Source: CAD feature listing. Evaluate the final solid. Frame: model axes, mm. Face numbers are marked on the shaded views. A direction names the side the tool comes from. Round coordinates to 2 decimals unless told otherwise and drop trailing zeros. Loops run counter-clockwise (first coordinate to the right, second up) from the corner with the lowest first, then second, coordinate; pieces in that order, holes last. Notation, with made-up numbers: M 67,0.5 L 92,0.5 A26 ccw 92,30.5 Z; hole C 16,77 d3. An arc over 180 degrees is marked long. Answer as a JSON object with one key per item and string values.
Autodesk Inventor part; units mm, degrees
ref_plane "YZ Plane" through (0, 0, 0) normal (1, 0, 0) x (0, 1, 0)
ref_plane "XZ Plane" through (0, 0, 0) normal (0, 1, 0) x (-1, 0, 0)
ref_plane "XY Plane" through (0, 0, 0) normal (0, 0, 1) x (1, 0, 0)
sketch "Sketch1" plane through (0, 0, 0) normal (1, 0, 0) x (0, 1, 0)
  line L0 (0, 0) -> (2.696, 0)
  line L1 (2.696, 0) -> (2.696, 6.6)
  circle A0 centre (2.696, 6.6) radius 0.5
  line L2 (-0.5, 0.5) -> (0.5, 0.5)
  line L3 (0.5, 0.5) -> (0.5, -0.5)
  line L4 (0.5, -0.5) -> (-0.5, -0.5)
  line L5 (-0.5, -0.5) -> (-0.5, 0.5)
  line L6 (-0.5, 0.5) -> (0.5, -0.5) construction
  line L7 (0.5, 0.5) -> (-0.5, -0.5) construction
  line L8 (0.5, -0.5) -> (3.1627, 6.4205)
  line L9 (-0.5, 0.5) -> (2.2374, 6.7993)
  dimension "d0" = 2.696
  dimension "d1" = 6.6
  dimension "d2" = 1
  dimension "d3" = 1
  dimension "d4" = 1
extrude "Extrusion1" add sketch "Sketch1" along normal blind 1 contours L3 L2 L9 A0 L1 L8 L0 | L3 L4 L5 L2 | L0 L8 L3 | L1 A0 L8 | A0
sketch "Sketch2" plane through (0, 0, 0) normal (-1, 0, 0) x (0, 0, 1)
  line L0 (-0.5, -0.5) -> (0.5, -0.5)
  line L1 (0.5, -0.5) -> (0.5, 0.5)
  line L2 (0.5, 0.5) -> (-0.5, 0.5)
  line L3 (-0.5, 0.5) -> (-0.5, -0.5)
  line L4 (-0.5, -0.5) -> (0.5, 0.5) construction
  line L5 (0.5, -0.5) -> (-0.5, 0.5) construction
  arc A0 (6.7993, 2.2374) -> (6.4205, 3.1627) centre (6.6, 2.696) ccw
  circle A1 centre (6.6, 2.696) radius 0.5
  point P0 (0, 0)
  point P1 (6.4205, 3.1627)
  point P2 (6.7993, 2.2374)
  dimension "d7" = 1
  dimension "d8" = 1
extrude "Extrusion2" add sketch "Sketch2" along normal blind 9.53
sketch "Sketch3" plane through (0, 3.1627, 6.4205) normal (0, 0.9333, -0.3591) x (1, 0, 0)
  line L0 (0, 0) -> (1, 0)
  line L1 (1, 0) -> (1, 4)
  line L2 (1, 7.415) -> (1, 0)
  line L3 (1, 4) -> (0, 4)
  circle A0 centre (0.5, 4) radius 0.5
  line L4 (1, 4) -> (1.9656, 2.6006)
  line L5 (1.9656, 2.6006) -> (1.9656, -0.469)
  line L6 (1.9656, -0.469) -> (1.3988, -1.3966)
  line L7 (1.3988, -1.3966) -> (-6.1023, -1.6689)
  line L8 (-6.1023, -1.6689) -> (-10.3351, -1.4334)
  line L9 (-10.3351, -1.4334) -> (-10.659, 1.386)
  line L10 (-10.659, 1.386) -> (-5.3662, 3.1822)
  line L11 (-5.3662, 3.1822) -> (0, 4)
  point P0 (0, 7.1279)
  point P1 (1, 4)
  dimension "d11" = 4
extrude "Extrusion3" cut sketch "Sketch3" against normal blind 10 contours L4 L5 L6 L7 L8 L9 L10 L11 A0
properties part number "Radius_Bone1_Joint_LOWER"
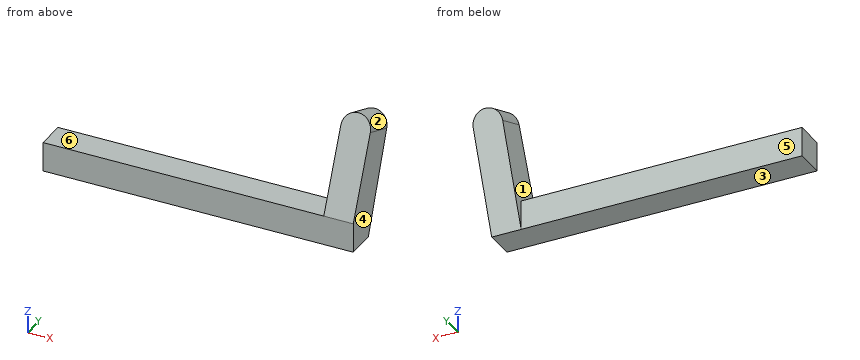
Item 1: Section D-D on z = 1.8. Return the cut outline in (x, y), then the cut area to 3 significant figures.
Answer sheet:
{"outline": "M 0,0.06 L 1,0.06 L 1,1.38 L 0,1.38 Z", "area": "1.32 mm²"}
Item 2: Access query for the marked faces 4, 5 and 6. Directions: +Z, -Z, +X, -X, +Y, -Y. A direction counts if a zero-diameter tool reaches every point of the face in a straight line with its end or side. Return the directions, or none.
Answer sheet:
{"face 4": "+Z, -Z, +X, +Y, -Y", "face 5": "+Z, -Z, -X, +Y", "face 6": "+Z, -X, +Y, -Y"}
Item 3: Contact query for a flat-ended pin moving along its axis: pin 1 Ø0.5 at (x, z) = (-4, 0) entering from +Y. Output: stop coordinate, or through.
Answer sheet:
{"pin 1": "stops at y = 0.5"}
Item 4: Section C-C on y = 0.25. Return the cut outline in (x, z), then the cut area to 3 significant figures.
Answer sheet:
{"outline": "M -9.53,-0.5 L 1,-0.5 L 1,2.23 L 0,2.23 L 0,0.5 L -9.53,0.5 Z", "area": "12.3 mm²"}
Item 5: Section A-A on x = -7.75. Return the cut outline in (y, z).
Answer sheet:
{"outline": "M -0.5,-0.5 L 0.5,-0.5 L 0.5,0.5 L -0.5,0.5 Z"}
Item 6: Section B-B on z = -0.2. Return the cut outline in (x, y).
Answer sheet:
{"outline": "M -9.53,-0.5 L 1,-0.5 L 1,0.62 L 0,0.62 L 0,0.5 L -9.53,0.5 Z"}
Item 7: Line query: probe 1 along Z at (x, y) = (-4.75, -0.2); probe 2 along X at (y, z) = (0.6, 0.4). Output: solid intervals per line, ascending. Write a range as from..to.
Answer sheet:
{"probe 1": "z = -0.5..0.5", "probe 2": "x = 0..1"}
Item 8: Pull-direction query (Z, two-part tool) for the marked faces 1, 2 and 3; classes: pulls with the +Z half, pulls with the -Z half, needs draft (parallel to the pull), parting line crosses it, or undercut.
Answer sheet:
{"face 1": "needs draft", "face 2": "pulls with the +Z half", "face 3": "pulls with the -Z half"}
